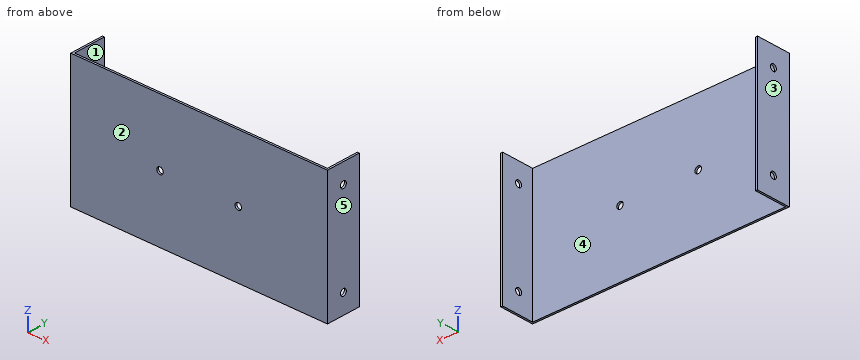
from build123d import *

# Parameters (mm, degrees)
SKETCH1_W           = 394
SKETCH1_H           = 200
BOSS_EXTRUDE1_DEPTH = 3
SKETCH2_W           = 3
SKETCH2_H           = 200
BOSS_EXTRUDE2_DEPTH = 50
SKETCH3_R           = 5
CUT_EXTRUDE1_DEPTH  = 410.932921342
SKETCH4_R           = 5
CUT_EXTRUDE2_DEPTH  = 228.195950668


with BuildPart() as part:
    # Sketch1 → Boss-Extrude1 (new body)
    with BuildSketch(Plane(origin=(0, 0, 0), x_dir=(1, 0, 0), z_dir=(0, 1, 0))):
        Rectangle(SKETCH1_W, SKETCH1_H)
    extrude(amount=BOSS_EXTRUDE1_DEPTH)

    # Sketch2 → Boss-Extrude2 (add)
    with BuildSketch(Plane(origin=(0, 3, 0), x_dir=(1, 0, 0), z_dir=(0, 1, 0))):
        with Locations((-195.5, 0)):
            Rectangle(SKETCH2_W, SKETCH2_H)
        with Locations((195.5, 0)):
            Rectangle(SKETCH2_W, SKETCH2_H)
    extrude(amount=BOSS_EXTRUDE2_DEPTH)

    # Sketch3 → Cut-Extrude1 (cut, through all)
    with BuildSketch(Plane(origin=(197, 0, 0), x_dir=(0, 0, -1), z_dir=(1, 0, 0))):
        with Locations((70, 26.5)):
            Circle(SKETCH3_R)
        with Locations((-70, 26.5)):
            Circle(SKETCH3_R)
    extrude(amount=-CUT_EXTRUDE1_DEPTH, mode=Mode.SUBTRACT)

    # Sketch4 → Cut-Extrude2 (cut, through all)
    with BuildSketch(Plane.XZ):
        with Locations(Location((60, 0, 0), (0, 0, 270))):
            Circle(SKETCH4_R)
        with Locations(Location((-60, 0, 0), (0, 0, 270))):
            Circle(SKETCH4_R)
    extrude(amount=-CUT_EXTRUDE2_DEPTH, mode=Mode.SUBTRACT)


solid = part.part
Read the model definition and answer for the solid it produces. Units are mm, in the model's axes. Face numbers are marked on the shaded views. A direction names the side the tool comes from. Give positions to 0.01 mm unless a question says otherwise; leave off trailing zeros. Loops run counter-clockwise (first coordinate to the right, second up) from the corner with the lowest first, then second, coordinate; pieces in that order, holes last. Notation, with made-up numbers: (19, -0.75) -> (75, -0.75) arc R25 ccw to (75, 30.25) -> close; hole circle Ø4 at (-11, 39.25). An arc over 180 degrees is marked (long way). Use a Markdown table: item, result.
Q1. Find the intervals of material crossed by line 1 along X through (y, z) = (50, -85); line 2 along Y through (x, z) = (111.5, 62), in increasing order.
Solved:
| item | result |
|---|---|
| line 1 | x = -197 to -194, 194 to 197 |
| line 2 | y = 0 to 3 |
Q2. Section A-A, the plane y = 36.5 is taken. Determine the outline of the cut face in (x, z), then the cut area to 3 significant figures.
Solved:
| item | result |
|---|---|
| outline | (-197, -100) -> (-194, -100) -> (-194, 100) -> (-197, 100) -> close; (194, -100) -> (197, -100) -> (197, 100) -> (194, 100) -> close |
| area | 1,200 mm^2 |
Q3. Section D-D, the plane z = -58 is taken. Determine the outline of the cut face in (x, y).
Solved:
| item | result |
|---|---|
| outline | (-197, 0) -> (197, 0) -> (197, 53) -> (194, 53) -> (194, 3) -> (-194, 3) -> (-194, 53) -> (-197, 53) -> close |
Q4. Each of these flat-tipped pins is pushed along its axis until it touches: pin 1 (13 mm diameter, centred on x = -60, z = 0, fed in from +Y); pin 2 (9 mm diameter, centred on y = 26.5, z = -70, fed in from +X). Where does it stop, or does it pass through?
Solved:
| item | result |
|---|---|
| pin 1 | stops at y = 3 |
| pin 2 | passes through |
Q5. A tool of negligible diameter and unlimited length cuts with its end or side. For the marked faces 4 and 5, from which of +Z, -Z, +X, -X, +Y, -Y can it reach the whole face along a straight path? Write none if from no direction.
Solved:
| item | result |
|---|---|
| face 4 | +Z, -Z, +Y |
| face 5 | +Z, -Z, +X, +Y, -Y |
Q6. Section B-B, the plane z = 70 is taken. Determine the outline of the cut face in (x, y).
Solved:
| item | result |
|---|---|
| outline | (-197, 0) -> (197, 0) -> (197, 21.5) -> (194, 21.5) -> (194, 3) -> (-194, 3) -> (-194, 21.5) -> (-197, 21.5) -> close; (-197, 31.5) -> (-194, 31.5) -> (-194, 53) -> (-197, 53) -> close; (194, 31.5) -> (197, 31.5) -> (197, 53) -> (194, 53) -> close |
Q7. Section C-C, the plane x = -60 is taken. Determine the outline of the cut face in (y, z).
Solved:
| item | result |
|---|---|
| outline | (0, -100) -> (3, -100) -> (3, -5) -> (0, -5) -> close; (0, 5) -> (3, 5) -> (3, 100) -> (0, 100) -> close |
Q8. Determine the mould class of the marked faces 1, 2 and 3 for opening direction X: pulls with the +X half, pulls with the -X half, needs draft (parallel to the pull), parting line crosses it, or undercut.
Solved:
| item | result |
|---|---|
| face 1 | undercut |
| face 2 | needs draft |
| face 3 | pulls with the -X half |
